```python
from build123d import *

# Parameters (mm, degrees)
EXTRUDE_2_DEPTH     = 18
EXTRUDE_3_DEPTH     = 30
SKETCH_1_8_R        = 10
SKETCH_1_8_R_2      = 5
EXTRUDE_4_DEPTH     = 40
EXTRUDE_5_DEPTH     = 36
CUT_EXTRUDE_1_DEPTH = 109


with BuildPart() as part:
    # Sketch 1 → Extrude 2 (new body)
    with BuildSketch(Plane.XY):
        with BuildLine():
            Line((0, 92), (0, 0))
            Line((0, 0), (10, 0))
            Line((10, 0), (10, 22))
            ThreePointArc((10, 22), (19, 31), (28, 22))
            Line((28, 22), (28, 0))
            Line((28, 0), (51, 0))
            Line((51, 0), (51, 92))
            Line((51, 92), (0, 92))
        make_face()
        with BuildLine():
            Line((40, 52.460607986), (34, 52.460607986))
            Line((34, 52.460607986), (34, 62.460607986))
            ThreePointArc((34, 62.460607986), (31.083920217, 80.062257748), (47, 72))
            ThreePointArc((47, 72), (45.062257748, 66.083920217), (40, 62.460607986))
            Line((40, 62.460607986), (40, 52.460607986))
        make_face(mode=Mode.SUBTRACT)
    extrude(amount=EXTRUDE_2_DEPTH)

    # Sketch 1_6 → Extrude 3 (add)
    with BuildSketch(Plane.XY):
        with BuildLine():
            Line((10, 22), (10, 0))
            Line((10, 0), (13, 0))
            Line((13, 0), (13, 22))
            ThreePointArc((13, 22), (19, 28), (25, 22))
            Line((25, 22), (25, 0))
            Line((25, 0), (28, 0))
            Line((28, 0), (28, 22))
            ThreePointArc((28, 22), (19, 31), (10, 22))
        make_face()
    extrude(amount=EXTRUDE_3_DEPTH)

    # Sketch 1_8 → Extrude 4 (add)
    with BuildSketch(Plane.XY):
        with Locations(Location((37, 72, 0), (0, 0, 252.542396876))):
            Circle(SKETCH_1_8_R)
        with Locations((37, 72)):
            Circle(SKETCH_1_8_R_2, mode=Mode.SUBTRACT)
    extrude(amount=EXTRUDE_4_DEPTH)

    # Sketch 1_9 → Extrude 5 (add)
    with BuildSketch(Plane.XY):
        with BuildLine():
            Line((34, 62.460607986), (34, 52.460607986))
            Line((34, 52.460607986), (40, 52.460607986))
            Line((40, 52.460607986), (40, 62.460607986))
            ThreePointArc((40, 62.460607986), (37, 62), (34, 62.460607986))
        make_face()
    extrude(amount=EXTRUDE_5_DEPTH)

    # Sketch 3 → Cut-Extrude 1 (cut, through all)
    with BuildSketch(Plane(origin=(40, 0, 0), x_dir=(0, 0, -1), z_dir=(1, 0, 0))):
        Polygon((-36, 62.460607986), (-18, 52.460607986), (-36, 52.460607986), align=None)
    extrude(amount=-CUT_EXTRUDE_1_DEPTH, mode=Mode.SUBTRACT)


solid = part.part
```
The listing builds one solid part. Answer for the finished solid, in the listing's coordinates (mm). A direction names the side the tool comes from. Give positions to 0.01 mm unless a question says otherwise; leave off trailing zeros. Loops run counter-clockwise (first coordinate to the right, second up) from the corner with the lowest first, then second, coordinate; pieces in that order, holes last. Notation, with made-up numbers: M -30,63.5 L 25,63.5 A13 cw 25,71.5 Z; hole C -26.5,83.25 d5. An arc over 180 degrees is marked long. One line per item, written item: value.
Q1. A cutting plane is placed at A-A on z = 11. Determine the outline of the cut face in (x, y), then the cut area to 3 significant figures.
Working result:
outline: M 0,0 L 13,0 L 13,22 A6 cw 25,22 L 25,0 L 51,0 L 51,92 L 0,92 Z; hole C 37,72 d10
area: 4,290 mm^2
Q2. A cutting plane is placed at B-B on x = 37. Determine the outline of the cut face in (y, z), then the cut area to 3 significant figures.
Working result:
outline: M 0,0 L 67,0 L 67,40 L 62,40 L 62,36 L 62.46,36 L 52.46,18 L 0,18 Z; M 77,0 L 92,0 L 92,18 L 82,18 L 82,40 L 77,40 Z
area: 1,780 mm^2
Q3. A cutting plane is placed at C-C on z = 19. Determine the outline of the cut face in (x, y).
Working result:
outline: M 10,0 L 13,0 L 13,22 A6 cw 25,22 L 25,0 L 28,0 L 28,22 A9 ccw 10,22 Z; M 34,53.02 L 40,53.02 L 40,62.46 A10 ccw long 34,62.46 Z; hole C 37,72 d10
Q4. Find the intervals of material crossed by line 1 (Y direction, x = 37, z = 9); line 2 (X direction, y = 5.5, z = 4); line 3 (X direction, y = 14, z = 21), in increasing order. Write a range as from..to.
Working result:
line 1: y = 0..67, 77..92
line 2: x = 0..13, 25..51
line 3: x = 10..13, 25..28
Q5. For faces 4 (the face through (25, 47, 18)), 5 (the face through (34, 59, 25)), 6 (the face through (40, 60, 23)), determine the directions among +Z, -Z, +X, -X, +Y, -Y from which every point of the face is accessible in a straight line to the end or side of a thin tool.
Working result:
face 4: +Z
face 5: +Z, -X, -Y
face 6: +Z, +X, -Y
Q6. Determine the mould class of faces 1 (the face through (0, 47, 9)), 2 (the face through (32, 72, 20)), 3 (the face through (38, 0, 8)) for opening direction X: +X half, -X half, draft (parallel to the pull), parting line (faces both ways), or undercut.
Working result:
face 1: -X half
face 2: undercut
face 3: draft
Q7. A cutting plane is placed at D-D on y = 69. Determine the outline of the cut face in (x, z), then the cut area to 3 significant figures.
Working result:
outline: M 0,0 L 33,0 L 33,40 L 27.46,40 L 27.46,18 L 0,18 Z; M 41,0 L 51,0 L 51,18 L 46.54,18 L 46.54,40 L 41,40 Z
area: 1,020 mm^2
Q8. Flat-ended cylindrical pins translate along their axes: P1, Ø2, axis at x = 12, y = 45.5, coming from the +Z side; P2, Ø14.5, axis at x = 20, y = 13.5, coming from the +Z side; P3, Ø5, axis at y = 56.5, z = 29.5, coming from the -X side. Find the tip coordinate at first contact, or state that the pin passes through.
Working result:
P1: stops at z = 18
P2: stops at z = 30
P3: stops at x = 34
